from build123d import *

# Parameters (mm, degrees)
SKETCH1_R           = 4
SKETCH1_R_2         = 3.5
BOSS_EXTRUDE1_DEPTH = 3
SKETCH2_W           = 12
SKETCH2_H           = 12
BOSS_EXTRUDE2_DEPTH = 1
FILLET10_R          = 2
FILLET11_R          = 2


with BuildPart() as part:
    # Sketch1 → Boss-Extrude1 (new body)
    with BuildSketch(Plane(origin=(0, 0, 0), x_dir=(1, 0, 0), z_dir=(0, 1, 0))):
        with Locations(Location((0, 0, 0), (0, 0, 270))):
            Circle(SKETCH1_R)
        with Locations(Location((0, 0, 0), (0, 0, 270))):
            Circle(SKETCH1_R_2, mode=Mode.SUBTRACT)
    extrude(amount=BOSS_EXTRUDE1_DEPTH)

    # Sketch2 → Boss-Extrude2 (add)
    with BuildSketch(Plane.XZ):
        Rectangle(SKETCH2_W, SKETCH2_H)
    extrude(amount=BOSS_EXTRUDE2_DEPTH)

    # Fillet10
    fillet10_edges = [part.edges().sort_by_distance(p)[0] for p in [
        (6, -0.5, -6),
        (6, -0.5, 6),
        (-6, -0.5, 6),
        (-6, -0.5, -6),
    ]]
    fillet(fillet10_edges, radius=FILLET10_R)

    # Fillet11
    # the kernel refuses this fillet: 2 mm, written as the material it takes off along each edge
    with BuildSketch(Plane(origin=(-4, 0, 4), x_dir=(0, 0, 1), z_dir=(1, 0, 0))) as fillet11_piece_1:
        with BuildLine():
            CenterArc((0.267949192, 2), FILLET11_R, 270, 60)
            Line((2, 1), (2.034641016, 0.98))
            ThreePointArc((2.034641016, 0.98), (2.04, 0.5), (2.04, 0))
            Line((2.04, 0), (2, -0.04))
            Line((2, -0.04), (0.267949192, -0.04))
            Line((0.267949192, -0.04), (0.267949192, 0))
        make_face()
    revolve(axis=Axis((-4, 0, 4), (0, -1, 0)), revolution_arc=90, mode=Mode.SUBTRACT)
    with BuildSketch(Plane(origin=(-4, 0, 6), x_dir=(0, -1, 0), z_dir=(1, 0, 0))) as fillet11_piece_2:
        with BuildLine():
            CenterArc((2, 1.732050808), FILLET11_R, 180, 60)
            Line((0, 1.732050808), (-0.04, 1.732050808))
            Line((-0.04, 1.732050808), (-0.04, 0))
            Line((-0.04, 0), (0, -0.04))
            ThreePointArc((0, -0.04), (0.5, -0.04), (0.98, -0.034641016))
            Line((0.98, -0.034641016), (1, 0))
        make_face()
    extrude(amount=8, mode=Mode.SUBTRACT)
    with BuildSketch(Plane(origin=(4, 0, 4), x_dir=(0, 0, 1), z_dir=(-1, 0, 0))) as fillet11_piece_3:
        with BuildLine():
            CenterArc((0.267949192, -2), FILLET11_R, 30, 60)
            Line((2, -1), (2.034641016, -0.98))
            ThreePointArc((2.034641016, -0.98), (2.04, -0.5), (2.04, 0))
            Line((2.04, 0), (2, 0.04))
            Line((2, 0.04), (0.267949192, 0.04))
            Line((0.267949192, 0.04), (0.267949192, 0))
        make_face()
    revolve(axis=Axis((4, 0, 4), (0, 1, 0)), revolution_arc=90, mode=Mode.SUBTRACT)
    with BuildSketch(Plane(origin=(4, 0, -4), x_dir=(1, 0, 0), z_dir=(0, 0, 1))) as fillet11_piece_4:
        with BuildLine():
            CenterArc((0.267949192, -2), FILLET11_R, 30, 60)
            Line((2, -1), (2.034641016, -0.98))
            ThreePointArc((2.034641016, -0.98), (2.04, -0.5), (2.04, 0))
            Line((2.04, 0), (2, 0.04))
            Line((2, 0.04), (0.267949192, 0.04))
            Line((0.267949192, 0.04), (0.267949192, 0))
        make_face()
    revolve(axis=Axis((4, 0, -4), (0, 1, 0)), revolution_arc=90, mode=Mode.SUBTRACT)
    with BuildSketch(Plane(origin=(4, 0, -6), x_dir=(0, 0, 1), z_dir=(-1, 0, 0)), Plane(origin=(6, 0, 4), x_dir=(-1, 0, 0), z_dir=(0, 0, -1)), Plane(origin=(-6, 0, -4), x_dir=(1, 0, 0), z_dir=(0, 0, 1))) as fillet11_piece_5:
        with BuildLine():
            CenterArc((1.732050808, -2), FILLET11_R, 90, 60)
            Line((0, -1), (-0.034641016, -0.98))
            ThreePointArc((-0.034641016, -0.98), (-0.04, -0.5), (-0.04, 0))
            Line((-0.04, 0), (0, 0.04))
            Line((0, 0.04), (1.732050808, 0.04))
            Line((1.732050808, 0.04), (1.732050808, 0))
        make_face()
    extrude(amount=8, mode=Mode.SUBTRACT)
    with BuildSketch(Plane(origin=(-4, 0, -4), x_dir=(-1, 0, 0), z_dir=(0, 0, 1))) as fillet11_piece_6:
        with BuildLine():
            CenterArc((0.267949192, 2), FILLET11_R, 270, 60)
            Line((2, 1), (2.034641016, 0.98))
            ThreePointArc((2.034641016, 0.98), (2.04, 0.5), (2.04, 0))
            Line((2.04, 0), (2, -0.04))
            Line((2, -0.04), (0.267949192, -0.04))
            Line((0.267949192, -0.04), (0.267949192, 0))
        make_face()
    revolve(axis=Axis((-4, 0, -4), (0, -1, 0)), revolution_arc=90, mode=Mode.SUBTRACT)


solid = part.part
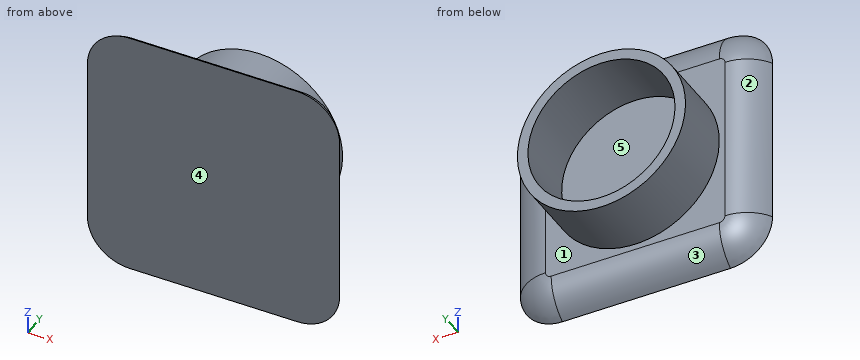
The listing builds one solid part. Answer for the finished solid, in the listing's coordinates (mm). Face numbers are marked on the shaded views. A direction names the side the tool comes from. Round coordinates to 2 decimals unless told otherwise and drop trailing zeros. Loops run counter-clockwise (first coordinate to the right, second up) from the corner with the lowest first, then second, coordinate; pieces in that order, holes last. Notation, with made-up numbers: M 15,79.5 L 40,79.5 A19 cw 40,92.5 Z; hole C -5.75,48.25 d3. An arc over 180 degrees is marked long. Return JSON: item names as keys, results as strings.
Q1. Find section C-C, the plane y = 1.8. Determine the outline of the cut face in (x, z).
Results list:
{"outline": "C 0,0 d8; hole C 0,0 d7"}
Q2. Which of the six approach directions +Z, -Z, +X, -X, +Y, -Y give full straight-line access (tool end or side, diameter ignored) to the marked faces 1 and 2?
Results list:
{"face 1": "+Y", "face 2": "+Z, -Z, -X, +Y"}
Q3. Find the intervals of material crossed by line 1 along Y through (x, z) = (-2, 4.25); line 2 along X through (y, z) = (1.3, 0); line 3 along X through (y, z) = (0.7, 1), in increasing order. Write a range as from..to.
Results list:
{"line 1": "y = -1..0", "line 2": "x = -4..-3.5, 3.5..4", "line 3": "x = -3.87..-3.35, 3.35..3.87"}
Q4. Find section B-B, the plane x = 0. Determine the outline of the cut face in (y, z).
Results list:
{"outline": "M -1,-6 A2 ccw 0,-4.27 L 0,-4 L 3,-4 L 3,-3.5 L 0,-3.5 L 0,3.5 L 3,3.5 L 3,4 L 0,4 L 0,4.27 A2 ccw -1,6 Z"}
Q5. The mould has two halves that part along Z. Classify the marked faces 3, 4 and 5: released by +Z, released by -Z, zero draft, split by the parting line, or undercut.
Results list:
{"face 3": "released by -Z", "face 4": "zero draft", "face 5": "undercut"}
Q6. Each of these flat-tipped pins is pushed along its axis until it touches: pin 1 Ø1.5 at (y, z) = (2.5, 3.5) entering from +X; pin 2 Ø2 at (x, z) = (-0.5, -1) entering from +Y; pin 3 Ø1 at (x, y) = (-3, 2.5) entering from +Z. Where does it stop, or does it pass through?
Results list:
{"pin 1": "stops at x = 2.9", "pin 2": "stops at y = 0", "pin 3": "stops at z = 3.12"}
Q7. Find section A-A, the plane z = 0. Determine the outline of the cut face in (x, y), plus the area to 3 significant figures.
Results list:
{"outline": "M -6,-1 L 6,-1 A2 ccw 4.27,0 L 4,0 L 4,3 L 3.5,3 L 3.5,0 L -3.5,0 L -3.5,3 L -4,3 L -4,0 L -4.27,0 A2 ccw Z", "area": "14.0 mm2"}
